Could you check a few things on this model? Use its own coordinates, in mm. Face numbers are marked on the shaded views. Round coordinates to 2 decimals unless told otherwise and drop trailing zeros. Write each loop counter-clockwise with the first axis right and the second up, starting at its lowest first coordinate (ties: lowest second). Pieces come first, ordered by that corner, then holes. Notation, with made-up numbers: (89, 39.5) -> (111, 39.5) arc R16 ccw to (111, 70.5) -> close; hole circle Ø4 at (82, -12). An arc over 180 degrees is marked (long way). Answer in a Markdown table with one row per item. Add a question column.
```python
from build123d import *

# Parameters (mm, degrees)
SKETCH1_R           = 50
BOSS_EXTRUDE1_DEPTH = 3
SKETCH2_R           = 50
SKETCH2_R_2         = 47
BOSS_EXTRUDE2_DEPTH = 4
SKETCH3_R           = 2
BOSS_EXTRUDE3_DEPTH = 27
CHAMFER1_SIZE       = 8
SKETCH4_R           = 46
SKETCH4_R_2         = 36
BOSS_EXTRUDE4_DEPTH = 2
CUT_EXTRUDE1_START  = 80
SKETCH5_W           = 25
SKETCH5_H           = 8
CUT_EXTRUDE1_DEPTH  = 59
CUT_EXTRUDE2_DEPTH  = 10
CUT_EXTRUDE3_DEPTH  = 10


with BuildPart() as part:
    # Sketch1 → Boss-Extrude1 (new body)
    with BuildSketch(Plane(origin=(0, 0, 0), x_dir=(1, 0, 0), z_dir=(0, 1, 0))):
        Circle(SKETCH1_R)
    extrude(amount=BOSS_EXTRUDE1_DEPTH)

    # Sketch2 → Boss-Extrude2 (add)
    with BuildSketch(Plane(origin=(0, 3, 0), x_dir=(1, 0, 0), z_dir=(0, 1, 0))):
        Circle(SKETCH2_R)
        Circle(SKETCH2_R_2, mode=Mode.SUBTRACT)
    extrude(amount=BOSS_EXTRUDE2_DEPTH)

    # Sketch3 → Boss-Extrude3 (add)
    with BuildSketch(Plane(origin=(0, 3, 0), x_dir=(1, 0, 0), z_dir=(0, 1, 0))):
        Circle(SKETCH3_R)
    extrude(amount=BOSS_EXTRUDE3_DEPTH)

    # Chamfer1
    chamfer1_edges = [part.edges().sort_by_distance(p)[0] for p in [
        (-2, 3, 0),
    ]]
    chamfer(chamfer1_edges, length=CHAMFER1_SIZE)

    # Sketch4 → Boss-Extrude4 (add)
    with BuildSketch(Plane(origin=(0, 3, 0), x_dir=(1, 0, 0), z_dir=(0, 1, 0))):
        Circle(SKETCH4_R)
        Circle(SKETCH4_R_2, mode=Mode.SUBTRACT)
    extrude(amount=BOSS_EXTRUDE4_DEPTH)

    # Sketch5 → Cut-Extrude1 (cut)
    with BuildSketch(Plane(origin=(0, 0, 0), x_dir=(0, 0, -1), z_dir=(1, 0, 0)).offset(CUT_EXTRUDE1_START)):
        with Locations((0, 7)):
            Rectangle(SKETCH5_W, SKETCH5_H)
    extrude(amount=-CUT_EXTRUDE1_DEPTH, mode=Mode.SUBTRACT)

    # Sketch7 → Cut-Extrude2 (cut)
    with BuildSketch(Plane.XZ):
        with BuildLine():
            Line((-119.395726794, 97.143761629), (-5.083168687, 49.740942855))
            ThreePointArc((-5.083168687, 49.740942855), (19.152450403, 46.186401067), (38.791481396, 31.547123024))
            Line((38.791481396, 31.547123024), (134.629479077, -8.194715589))
            Line((134.629479077, -8.194715589), (149.847747334, 28.504350406))
            Line((149.847747334, 28.504350406), (-104.177458536, 133.842827624))
            Line((-104.177458536, 133.842827624), (-119.395726794, 97.143761629))
        make_face()
        with BuildLine():
            ThreePointArc((38.791481396, 31.547123024), (41.025780027, 28.581206642), (43.033800963, 25.457650612))
            Line((43.033800963, 25.457650612), (133.097283044, -11.889627674))
            Line((133.097283044, -11.889627674), (134.629479077, -8.194715589))
            Line((134.629479077, -8.194715589), (38.791481396, 31.547123024))
        make_face()
        with BuildLine():
            ThreePointArc((38.791481396, 31.547123024), (19.152450403, 46.186401067), (-5.083168687, 49.740942855))
            Line((-5.083168687, 49.740942855), (38.791481396, 31.547123024))
        make_face()
        with BuildLine():
            ThreePointArc((-5.083168687, 49.740942855), (-8.76068428, 49.226521418), (-12.389880318, 48.440591096))
            Line((-12.389880318, 48.440591096), (43.033800963, 25.457650612))
            ThreePointArc((43.033800963, 25.457650612), (41.025780027, 28.581206642), (38.791481396, 31.547123024))
            Line((38.791481396, 31.547123024), (-5.083168687, 49.740942855))
        make_face()
        with BuildLine():
            Line((-120.927922826, 93.448849543), (-12.389880318, 48.440591096))
            ThreePointArc((-12.389880318, 48.440591096), (-8.76068428, 49.226521418), (-5.083168687, 49.740942855))
            Line((-5.083168687, 49.740942855), (-119.395726794, 97.143761629))
            Line((-119.395726794, 97.143761629), (-120.927922826, 93.448849543))
        make_face()
        with BuildLine():
            Line((-11.858515668, -55.706448378), (84.665757499, -95.732869831))
            Line((84.665757499, -95.732869831), (92.00979772, -81.45716056))
            Line((92.00979772, -81.45716056), (86.695290109, -79.253355087))
            Line((86.695290109, -79.253355087), (87.844437133, -76.482171023))
            Line((87.844437133, -76.482171023), (16.892477306, -47.060006486))
            ThreePointArc((16.892477306, -47.060006486), (-19.152450403, -46.186401067), (-45.238103903, -21.295867094))
            Line((-45.238103903, -21.295867094), (-140.17236541, 18.071212676))
            Line((-140.17236541, 18.071212676), (-142.248536864, 13.06449628))
            Line((-142.248536864, 13.06449628), (-142.248536864, 11.37179915))
            Line((-142.248536864, 11.37179915), (-11.858515668, -55.706448378))
        make_face()
        with BuildLine():
            ThreePointArc((-45.238103903, -21.295867094), (-19.152450403, -46.186401067), (16.892477306, -47.060006486))
            Line((16.892477306, -47.060006486), (-45.238103903, -21.295867094))
        make_face()
    extrude(amount=-CUT_EXTRUDE2_DEPTH, mode=Mode.SUBTRACT)

    # Sketch8 → Cut-Extrude3 (cut)
    with BuildSketch(Plane.XZ):
        with BuildLine():
            ThreePointArc((16.892477306, -47.060006486), (18.883795364, -46.296892689), (20.840762361, -45.44956132))
            Line((20.840762361, -45.44956132), (18.04162433, -44.288822422))
            Line((18.04162433, -44.288822422), (-44.088956879, -18.52468303))
            Line((-44.088956879, -18.52468303), (-46.888094909, -17.363944131))
            ThreePointArc((-46.888094909, -17.363944131), (-46.105033689, -19.347502903), (-45.238103903, -21.295867094))
            Line((-45.238103903, -21.295867094), (16.892477306, -47.060006486))
        make_face()
        with BuildLine():
            Line((41.387159819, 22.892766048), (41.884653939, 22.686466548))
            Line((41.884653939, 22.686466548), (45.238103903, 21.295867094))
            ThreePointArc((45.238103903, 21.295867094), (44.184979435, 23.402726173), (43.033800963, 25.457650612))
            Line((43.033800963, 25.457650612), (-12.389880318, 48.440591096))
            ThreePointArc((-12.389880318, 48.440591096), (-14.657442494, 47.803340673), (-16.892477306, 47.060006486))
            Line((-16.892477306, 47.060006486), (-13.539027342, 45.669407032))
            Line((-13.539027342, 45.669407032), (-11.390013124, 44.778259697))
            Line((-11.390013124, 44.778259697), (41.387159819, 22.892766048))
        make_face()
    extrude(amount=-CUT_EXTRUDE3_DEPTH, mode=Mode.SUBTRACT)


solid = part.part
```
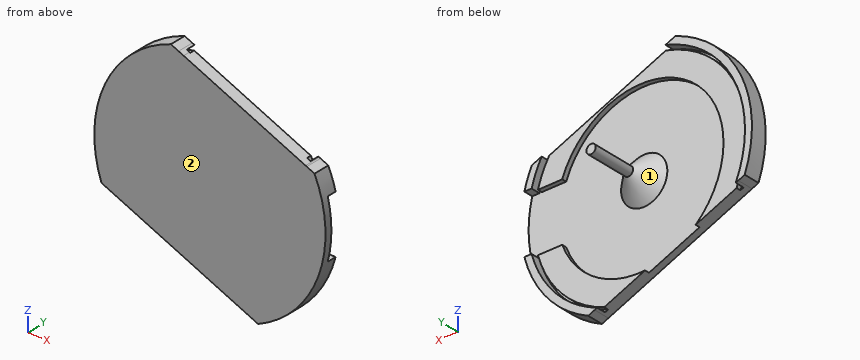
(1) Suppose I cut it at D-D, the plane z = 38. Please give me the cut outline in (x, y).
(2) Suppose I cut it at B-B, the plane x = 0. Please give me the cut outline in (y, z), then the cut area to 3 significant figures.
(3) For P1, Ø0.9, axis at x = 46.5, y = 5, coming from the +Z side; P2, Ø3.5, axis at x = 43.5, z = 17.5, coming from the +Y side; P3, Ø3, axis at x = 26.5, z = 2, coming from the -Y side; P4, Ø3.5, axis at x = 46.5, y = 4, coming from the -Z side, each with a flat end and sliding along its axis, tell me the tip position at first contact or that it passes through.
(4) Suppose I cut it at C-C, the plane y = 25.5. Please give me the cut outline in (x, z), then the cut area to 3 significant figures.
(5) I need wall thicknesses on L1, parallel to Z at x = 0, y = 4.05; L2, parallel to X at y = 3.95, z = 0; L3, parallel to X at y = 4.4, z = 0. Which ranges of each line are inside material? Lowest first, please.
(6) Suppose I cut it at A-A, the plane z = 0. Please give me the cut outline in (x, y).
(7) If we mould it in two halves opening along Z, with no side actions, what happens to the marked faces 1 and 2? For each: pulls with the +Z half, pulls with the -Z half, needs draft (parallel to the pull), parting line crosses it, or undercut.
Response:
| question | item | result |
|---|---|---|
| 1 | outline | (-32.5, 0) -> (4.96, 0) -> (4.96, 5) -> (-25.92, 5) -> (-25.92, 3) -> (-27.66, 3) -> (-27.66, 7) -> (-32.5, 7) -> close |
| 2 | outline | (0, -36.81) -> (5, -36.81) -> (5, -36) -> (3, -36) -> (3, -10) -> (11, -2) -> (30, -2) -> (30, 2) -> (11, 2) -> (3, 10) -> (3, 36) -> (5, 36) -> (5, 40.06) -> (0, 40.06) -> close |
| 2 | area | 412 mm² |
| 3 | P1 | z = 19.48 |
| 3 | P2 | y = 7 |
| 3 | P3 | y = 0 |
| 3 | P4 | z = -22.3 |
| 4 | outline | circle Ø4 at (0, 0) |
| 4 | area | 12.6 mm² |
| 5 | L1 | -36.81 to -36, -8.95 to 8.95, 36 to 40.06 |
| 5 | L2 | -50 to -47, -46 to -36, -9.05 to 9.05 |
| 5 | L3 | -50 to -47, -46 to -36, -8.6 to 8.6 |
| 6 | outline | (-50, 0) -> (50, 0) -> (50, 3) -> (10, 3) -> (2, 11) -> (2, 30) -> (-2, 30) -> (-2, 11) -> (-10, 3) -> (-36, 3) -> (-36, 5) -> (-46, 5) -> (-46, 3) -> (-47, 3) -> (-47, 7) -> (-50, 7) -> close |
| 7 | face 1 | undercut |
| 7 | face 2 | needs draft |
